```python
from build123d import *

# Parameters (mm, degrees)
SKETCH1_R               = 23.75
SKETCH1_R_2             = 21.75
BOSS_EXTRUDE1_DEPTH     = 59
SKETCH2_R               = 23.75
BOSS_EXTRUDE2_DEPTH     = 2
SKETCH3_R               = 1.5
CUT_EXTRUDE1_DEPTH      = 2
CUT_EXTRUDE2_REACH      = 71.636
CUT_EXTRUDE2_END_RADIUS = 23.75
SKETCH4_R               = 2
CIRPATTERN1_COUNT       = 3


with BuildPart() as part:
    # Sketch1 → Boss-Extrude1 (new body)
    with BuildSketch(Plane(origin=(0, 0, 0), x_dir=(1, 0, 0), z_dir=(0, 1, 0))):
        with Locations(Location((0, 0, 0), (0, 0, 270))):
            Circle(SKETCH1_R)
        with Locations(Location((0, 0, 0), (0, 0, 270))):
            Circle(SKETCH1_R_2, mode=Mode.SUBTRACT)
    extrude(amount=BOSS_EXTRUDE1_DEPTH)

    # Sketch2 → Boss-Extrude2 (add)
    with BuildSketch(Plane(origin=(0, 59, 0), x_dir=(1, 0, 0), z_dir=(0, 1, 0))):
        with Locations(Location((0, 0, 0), (0, 0, 270))):
            Circle(SKETCH2_R)
    extrude(amount=BOSS_EXTRUDE2_DEPTH)

    # Sketch3 → Cut-Extrude1 (cut)
    with BuildSketch(Plane(origin=(0, 61, 0), x_dir=(1, 0, 0), z_dir=(0, 1, 0))):
        with Locations(Location((-10.5, 0, 0), (0, 0, 270))):
            Circle(SKETCH3_R)
        with Locations(Location((10.5, 0, 0), (0, 0, 270))):
            Circle(SKETCH3_R)
        with Locations(Location((-10.5, -12.5, 0), (0, 0, 270))):
            Circle(SKETCH3_R)
        with Locations(Location((10.5, -12.5, 0), (0, 0, 270))):
            Circle(SKETCH3_R)
        Polygon((0, 7.4), (6.8, 7.4), (6.8, -15.6), (-6.94269124, -15.6), (-6.94269124, 7.4), align=None)
    extrude(amount=-CUT_EXTRUDE1_DEPTH, mode=Mode.SUBTRACT)

    # Cut-Extrude2: up to this cylinder (the profile starts inside it)
    cut_extrude2_end = Plane(origin=(0, 10, 0), z_dir=(0, -1, 0)) * Cylinder(CUT_EXTRUDE2_END_RADIUS, 191.772, mode=Mode.PRIVATE)
    # Sketch4 → Cut-Extrude2 (cut, up to the surface)
    with BuildSketch(Plane.XY, mode=Mode.PRIVATE) as cut_extrude2_sk1:
        with Locations((0, 10)):
            Circle(SKETCH4_R)
    cut_extrude2_tool1 = extrude(cut_extrude2_sk1.sketch, amount=-CUT_EXTRUDE2_REACH, mode=Mode.PRIVATE) & cut_extrude2_end
    cut_extrude2 = cut_extrude2_tool1.solids().sort_by_distance((0, 10, 0))[0]
    add(cut_extrude2, mode=Mode.SUBTRACT)

    # CirPattern1: Cut-Extrude2 ×3 about axis
    cirpattern1_axis = Axis((0, 59, 0), (0, -1, 0))
    for i in range(1, CIRPATTERN1_COUNT):
        add(cut_extrude2.rotate(cirpattern1_axis, i * 360 / CIRPATTERN1_COUNT), mode=Mode.SUBTRACT)


solid = part.part
```
Can you work these out from the model? Positions are in its coordinate system, mm. A direction names the side the tool comes from. Round coordinates to 2 decimals unless told otherwise and drop trailing zeros. Loops run counter-clockwise (first coordinate to the right, second up) from the corner with the lowest first, then second, coordinate; pieces in that order, holes last.
Item 1: Which directions (+Z, -Z, +X, -X, +Y, -Y) give clear straight access to the entire face, cutting with the end or side of a thin tool? Please do faces 1 (the cylindrical face through (-20.186, 11.686, 10.413)), 2 (the cylindrical face through (21.565, 29.087, -2.831)), 3 (the flat face through (-6.943, 60, 4)), 4 (the cylindrical face through (0, 12, -23)), 5 (the flat face through (0, 61, -11)).
Item 2: Suppose I cut it at D-D, the plane y = 10. Write out the boundary of the cut face in (x, z).
Item 3: Suppose I cut it at A-A, the plane z = 0. Write out the boundary of the cut face in (x, y).
Item 4: Will these pins go through, and if not, where does the flat tip stop? pin 1 Ø8 at (x, z) = (-10.5, -0.5) entering from -Y; pin 2 Ø4 at (y, z) = (43, 16) entering from +X; pin 3 Ø1.6 at (y, z) = (60, 7.5) entering from +X.
Item 5: If we mould it in two halves opening along X, with no side actions, what happens to faces 6 (the flat face through (0, 59, -10)), 7 (the cylindrical face through (-23.185, 30.073, -5.149)), 8 (the flat face through (-7, 0, 21)), 9 (the flat face through (0, 60, -7.4))? For each: +X half, -X half, draft (parallel to the pull), parting line (faces both ways), or undercut.
Item 6: Please list where these lines run through material, in increasing order: L1, parallel to X at y = 60.2, z = 0; L2, parallel to Z at x = 0, y = 58.5; L3, parallel to X at y = 60, z = 12.
Item 7: Suppose I cut it at B-B, the plane x = 6. Write out the boundary of the cut face in (y, z).
Item 8: Suppose I cut it at C-C, the plane y = 54.5. Write out the boundary of the cut face in (x, z), then the cut area to 3 significant figures.
Reported:
1. face 1: none
1. face 2: -Y
1. face 3: +Y, -Y
1. face 4: -Z
1. face 5: +Z, -Z, +X, -X, +Y
2. outline: (-21.5, 10.1) arc R23.75 ccw to (-2, -23.67) - (-2, -21.66) arc R21.75 cw to (-19.76, 9.1) - close; (-19.5, 13.56) - (-17.76, 12.56) arc R21.75 cw to (17.76, 12.56) - (19.5, 13.56) arc R23.75 ccw to start; (2, -23.67) arc R23.75 ccw to (21.5, 10.1) - (19.76, 9.1) arc R21.75 cw to (2, -21.66) - close
3. outline: (-23.75, 0) - (-21.75, 0) - (-21.75, 59) - (-12, 59) - (-12, 61) - (-23.75, 61) - close; (-9, 59) - (-6.94, 59) - (-6.94, 61) - (-9, 61) - close; (6.8, 59) - (9, 59) - (9, 61) - (6.8, 61) - close; (12, 59) - (21.75, 59) - (21.75, 0) - (23.75, 0) - (23.75, 61) - (12, 61) - close
4. pin 1: stops at y = 59
4. pin 2: stops at x = 19.18
4. pin 3: stops at x = 22.79
5. face 6: undercut
5. face 7: parting line
5. face 8: draft
5. face 9: undercut
6. L1: x = -23.75 to -12, -9 to -6.94, 6.8 to 9, 12 to 23.75
6. L2: z = -23.75 to -21.75, 21.75 to 23.75
6. L3: x = -20.5 to -11.91, -9.09 to -6.94, 6.8 to 9.09, 11.91 to 20.5
7. outline: (0, -22.98) - (61, -22.98) - (61, -7.4) - (59, -7.4) - (59, -20.91) - (0, -20.91) - close; (0, 20.91) - (59, 20.91) - (59, 15.6) - (61, 15.6) - (61, 22.98) - (0, 22.98) - close
8. outline: circle Ø47.5 at (0, 0); hole circle Ø43.5 at (0, 0)
8. area: 286 mm2
